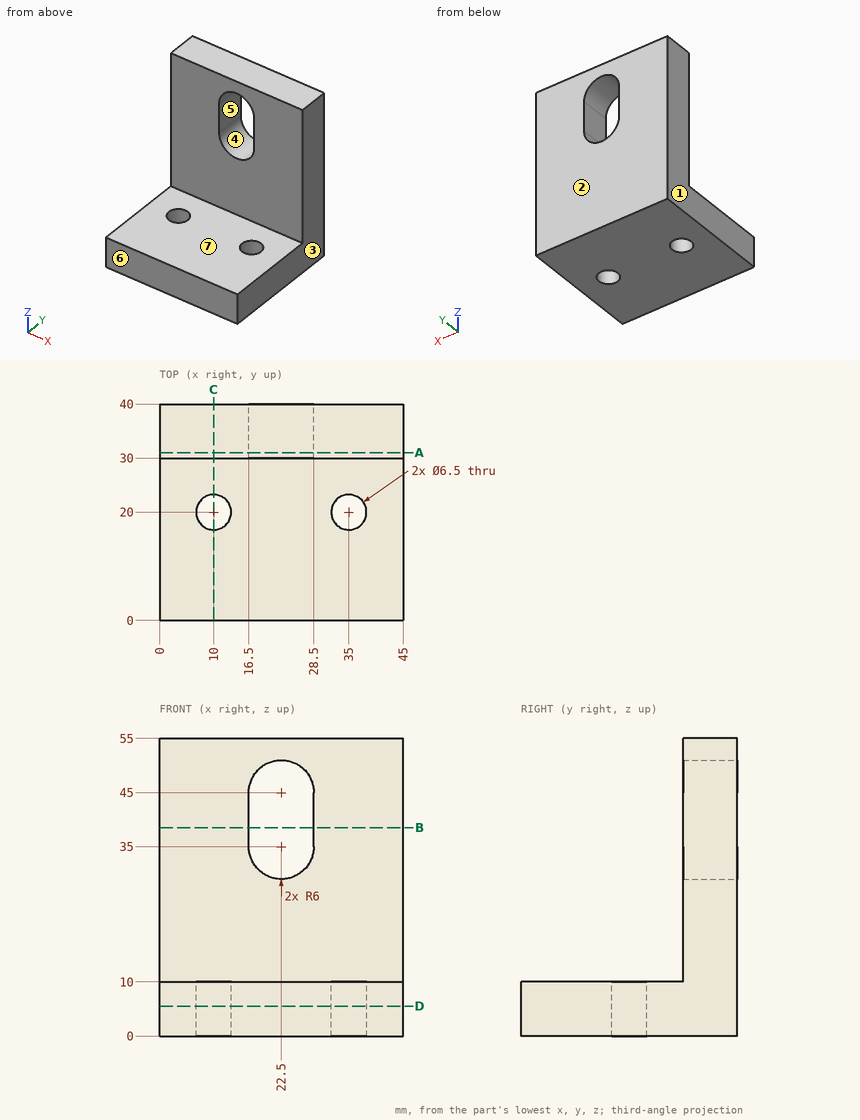
Print and shaded views of the part. All mm, measured from the part's lowest x, y and z. A direction names the side the tool comes from. Give positions to 0.01 mm unless a question says otherwise; leave off trailing zeros. Loops run counter-clockwise (first coordinate to the right, second up) from the corner with the lowest first, then second, coordinate; pieces in that order, holes last. Notation, with made-up numbers: (-32.5, 1.25) - (-19.5, 1.25) arc R25 cw to (-19.5, 20.25) - close; hole circle Ø11 at (89.25, -28.75). An arc over 180 degrees is marked (long way). One line per item, written item: value. Start each with the question number.
1. Slice it at C-C (x = 10). List the corners of the cut face in (y, z).
2. Slice it at B-B (z = 38.5). List the corners of the cut face in (x, y), plus the area to 3 significant figures.
3. Pull direction X, two halves, no side cores. Call the marked faces 1, 2, 3 and 4: pulls with the +X half, pulls with the -X half, needs draft (parallel to the pull), parting line crosses it, or undercut.
4. Slice it at D-D (z = 5.5). List the corners of the cut face in (x, y).
5. Probe L1, parallel to X at y = 20, z = 4.75; L2, parallel to X at y = 34, z = 44.5; L3, parallel to Y at x = 35, z = 4.5. List the from-to ranges inside material, lowest first. Write a range as from..to.
6. Pin check, flat tips, straight feed: pin 1 (3 mm diameter, centred on x = 37, y = 19.5, fed in from +Z); pin 2 (6 mm diameter, centred on x = 35, z = 43.5, fed in from -Y). Stop position of each tip, or through.
7. Slice it at A-A (y = 31). List the corners of the cut face in (x, z).
8. Which spindle directions (+Z, -Z, +X, -X, +Y, -Y) get a long thin tool onto all of the face, cutting with end or side? Do the marked faces 5, 6 and 7. Say none if no direction does.
Solution:
1. outline: (0, 0) - (16.75, 0) - (16.75, 10) - (0, 10) - close; (23.25, 0) - (40, 0) - (40, 55) - (30, 55) - (30, 10) - (23.25, 10) - close
2. outline: (0, 30) - (16.5, 30) - (16.5, 40) - (0, 40) - close; (28.5, 30) - (45, 30) - (45, 40) - (28.5, 40) - close
2. area: 330 mm^2
3. face 1: pulls with the -X half
3. face 2: needs draft
3. face 3: pulls with the +X half
3. face 4: undercut
4. outline: (0, 0) - (45, 0) - (45, 40) - (0, 40) - close; hole circle Ø6.5 at (10, 20); hole circle Ø6.5 at (35, 20)
5. L1: x = 0..6.75, 13.25..31.75, 38.25..45
5. L2: x = 0..16.5, 28.5..45
5. L3: y = 0..16.75, 23.25..40
6. pin 1: stops at z = 10
6. pin 2: stops at y = 30
7. outline: (0, 0) - (45, 0) - (45, 55) - (0, 55) - close; hole (16.5, 35) arc R6 ccw to (28.5, 35) - (28.5, 45) arc R6 ccw to (16.5, 45) - close
8. face 5: +Y, -Y
8. face 6: +Z, -Z, +X, -X, -Y
8. face 7: +Z, +X, -X, -Y
